Read the model definition and answer for the solid it produces. Units are mm, in the model's axes. A direction names the side the tool comes from. Give positions to 0.01 mm unless a question says otherwise; leave off trailing zeros. Order: outer loops, then holes, each group sorted by start corner. A loop starts at its lowest first (then second) coordinate and runs counter-clockwise, first axis right, second up. Notation, with made-up numbers: M 39.25,-7.5 L 72.25,-7.5 A12 cw 72.25,7.5 Z; hole C 1.5,-35 d2. An arc over 180 degrees is marked long. One line per item, written item: value.
from build123d import *

# Parameters (mm, degrees)
SKETCH1_R                       = 31.623
BOSS_EXTRUDE1_DEPTH             = 66.802
CUT_EXTRUDE1_START              = -10.668
CUT_EXTRUDE1_DEPTH              = 10.668
CHAMFER1_SIZE                   = 4.6355
SKETCH3_R                       = 10.2235
BOSS_EXTRUDE2_DEPTH             = 2.6289
SKETCH4_R                       = 4
BOSS_EXTRUDE3_DEPTH             = 2.032
SKETCH5_R                       = 8.7376
BOSS_EXTRUDE4_DEPTH             = 12.3698
BOSS_EXTRUDE5_START             = 27.686
SKETCH6_R                       = 4
BOSS_EXTRUDE5_DEPTH             = 27.686
M4X0_7_TAPPED_HOLE1_D           = 3.3
M4X0_7_TAPPED_HOLE1_DEPTH       = 9.906
M4X0_7_TAPPED_HOLE1_CSINK_D     = 4.05
M4X0_7_TAPPED_HOLE1_CSINK_ANGLE = 90
M4X0_7_TAPPED_HOLE1_TIP         = 0.991420021
FILLET1_R                       = 3.175


with BuildPart() as part:
    # Sketch1 → Boss-Extrude1 (new body)
    with BuildSketch(Plane(origin=(0, 0, 0), x_dir=(0, 0, -1), z_dir=(1, 0, 0))):
        Circle(SKETCH1_R)
    extrude(amount=BOSS_EXTRUDE1_DEPTH)

    # Sketch2 → Cut-Extrude1 (cut)
    with BuildSketch(Plane(origin=(66.802, 0, 0), x_dir=(0, 0, -1), z_dir=(1, 0, 0)).offset(CUT_EXTRUDE1_START)):
        with BuildLine():
            Line((-27.43403991, 15.728559476), (-12.052689417, 6.848132628))
            ThreePointArc((-12.052689417, 6.848132628), (-7.45361258, 7.45361258), (-6.848132628, 12.052689417))
            Line((-6.848132628, 12.052689417), (-15.728559476, 27.43403991))
            ThreePointArc((-15.728559476, 27.43403991), (-22.360837741, 22.360837741), (-27.43403991, 15.728559476))
        make_face()
        with BuildLine():
            ThreePointArc((-29.823578313, -10.515146485), (-20.955, 0), (-29.823578313, 10.515146485))
            ThreePointArc((-29.823578313, 10.515146485), (-31.623, 0), (-29.823578313, -10.515146485))
        make_face()
        with BuildLine():
            ThreePointArc((6.848132628, 12.052689417), (7.45361258, 7.45361258), (12.052689417, 6.848132628))
            Line((12.052689417, 6.848132628), (27.43403991, 15.728559476))
            ThreePointArc((27.43403991, 15.728559476), (22.360837741, 22.360837741), (15.728559476, 27.43403991))
            Line((15.728559476, 27.43403991), (6.848132628, 12.052689417))
        make_face()
        with BuildLine():
            ThreePointArc((-6.848132628, -12.052689417), (-7.45361258, -7.45361258), (-12.052689417, -6.848132628))
            Line((-12.052689417, -6.848132628), (-27.43403991, -15.728559476))
            ThreePointArc((-27.43403991, -15.728559476), (-22.360837741, -22.360837741), (-15.728559476, -27.43403991))
            Line((-15.728559476, -27.43403991), (-6.848132628, -12.052689417))
        make_face()
        with BuildLine():
            ThreePointArc((10.515146485, 29.823578313), (0, 31.623), (-10.515146485, 29.823578313))
            ThreePointArc((-10.515146485, 29.823578313), (0, 20.955), (10.515146485, 29.823578313))
        make_face()
        with BuildLine():
            ThreePointArc((12.052689417, -6.848132628), (7.45361258, -7.45361258), (6.848132628, -12.052689417))
            Line((6.848132628, -12.052689417), (15.728559476, -27.43403991))
            ThreePointArc((15.728559476, -27.43403991), (22.360837741, -22.360837741), (27.43403991, -15.728559476))
            Line((27.43403991, -15.728559476), (12.052689417, -6.848132628))
        make_face()
        with BuildLine():
            ThreePointArc((29.823578313, -10.515146485), (31.623, 0), (29.823578313, 10.515146485))
            ThreePointArc((29.823578313, 10.515146485), (20.955, 0), (29.823578313, -10.515146485))
        make_face()
        with BuildLine():
            ThreePointArc((10.515146485, -29.823578313), (0, -20.955), (-10.515146485, -29.823578313))
            ThreePointArc((-10.515146485, -29.823578313), (0, -31.623), (10.515146485, -29.823578313))
        make_face()
    extrude(amount=CUT_EXTRUDE1_DEPTH, mode=Mode.SUBTRACT)

    # Chamfer1
    chamfer1_edges = [part.edges().sort_by_distance(p)[0] for p in [
        (66.802, 13.176133693, -28.747236909),
        (66.802, 28.747236909, -13.176133693),
        (66.802, 28.747236909, 13.176133693),
        (66.802, 13.176133693, 28.747236909),
        (66.802, -13.176133693, 28.747236909),
        (66.802, -28.747236909, 13.176133693),
        (66.802, -28.747236909, -13.176133693),
        (66.802, -13.176133693, -28.747236909),
    ]]
    chamfer(chamfer1_edges, length=CHAMFER1_SIZE)

    # Sketch3 → Boss-Extrude2 (add)
    with BuildSketch(Plane(origin=(66.802, 0, 0), x_dir=(0, 0, -1), z_dir=(1, 0, 0))):
        Circle(SKETCH3_R)
    extrude(amount=BOSS_EXTRUDE2_DEPTH)

    # Sketch4 → Boss-Extrude3 (add)
    with BuildSketch(Plane(origin=(69.4309, 0, 0), x_dir=(0, 0, -1), z_dir=(1, 0, 0))):
        Circle(SKETCH4_R)
    extrude(amount=BOSS_EXTRUDE3_DEPTH)

    # Sketch5 → Boss-Extrude4 (add)
    with BuildSketch(Plane.ZY):
        Circle(SKETCH5_R)
    extrude(amount=BOSS_EXTRUDE4_DEPTH)

    # Sketch6 → Boss-Extrude5 (add)
    with BuildSketch(Plane.ZY.offset(12.3698).offset(BOSS_EXTRUDE5_START)):
        with Locations(Location((0, 0, 0), (0, 0, 180))):
            Circle(SKETCH6_R)
    extrude(amount=-BOSS_EXTRUDE5_DEPTH)

    # M4x0.7 Tapped Hole1
    with Locations(Plane.ZY):
        with Locations((0, 22.05), (-22.05, 0), (0, -22.05), (22.05, 0)):
            CounterSinkHole(M4X0_7_TAPPED_HOLE1_D / 2, M4X0_7_TAPPED_HOLE1_CSINK_D / 2, depth=M4X0_7_TAPPED_HOLE1_DEPTH, counter_sink_angle=M4X0_7_TAPPED_HOLE1_CSINK_ANGLE)
            with Locations((0, 0, -(M4X0_7_TAPPED_HOLE1_DEPTH + M4X0_7_TAPPED_HOLE1_TIP / 2))):  # 118° drill point
                Cone(0, M4X0_7_TAPPED_HOLE1_D / 2, M4X0_7_TAPPED_HOLE1_TIP, mode=Mode.SUBTRACT)

    # Fillet1
    fillet1_edges = [part.edges().sort_by_distance(p)[0] for p in [
        (0, 0, 31.623),
    ]]
    fillet(fillet1_edges, radius=FILLET1_R)


solid = part.part
1) Which of the six approach directions +Z, -Z, +X, -X, +Y, -Y give full straight-line access (tool end or side, diameter ignored) to faces 1 (the face through (56.134, 0, -26)), 2 (the face through (0, 7, -6)), 3 (the face through (66.802, 0, -11))?
Reported:
face 1: -Z, +X
face 2: -X
face 3: +X
2) Consider probe 1 along Y at (x, z) = (5, 0); probe 2 along X at (y, z) = (21, 15). Determine where each line is inside the solid, lowest interval first.
Reported:
probe 1: y = -31.62 to -23.7, -20.4 to 20.4, 23.7 to 31.62
probe 2: x = 0 to 56.13
3) Find section B-B, the plane x = -3.5. Write down the section's boundary in (y, z), plus the area to 3 significant figures.
Reported:
outline: C 0,0 d17.48
area: 240 mm^2
4) Determine the mould class of faces 4 (the face through (56.134, 17, -17)), 5 (the face through (-26.407, 3.905, 0.867)), 6 (the face through (56.134, 0, 26)) for opening direction Z: +Z half, -Z half, draft (parallel to the pull), parting line (faces both ways), or undercut.
Reported:
face 4: undercut
face 5: parting line
face 6: draft
5) Find section A-A, the plane x = 17. Write down the section's boundary in (y, z).
Reported:
outline: C 0,0 d63.25
6) Each of these flat-tipped pins is pushed along its axis until it touches: pin 1 Ø4 at (y, z) = (-22.05, 0) entering from +X; pin 2 Ø1 at (x, y) = (59.5, -18) entering from +Z; pin 3 Ø8.5 at (y, z) = (1.5, -27.5) entering from +X. Where does it stop, or does it pass through?
Reported:
pin 1: stops at x = 66.8
pin 2: stops at z = 10.57
pin 3: stops at x = 56.13
